Source: CAD feature listing. Evaluate the final solid. Frame: model axes, mm. A direction names the side the tool comes from. Give positions to 0.01 mm unless a question says otherwise; leave off trailing zeros. Loops run counter-clockwise (first coordinate to the right, second up) from the corner with the lowest first, then second, coordinate; pieces in that order, holes last. Notation, with made-up numbers: M -25,-9.5 L 3,-9.5 A21 ccw 3,14.5 Z; hole C -37.5,2 d4. An arc over 180 degrees is marked long. Write item = value, one per line.
Autodesk Inventor part; units mm, degrees
ref_plane "YZ Plane" through (0, 0, 0) normal (1, 0, 0) x (0, 1, 0)
ref_plane "XZ Plane" through (0, 0, 0) normal (0, 1, 0) x (-1, 0, 0)
ref_plane "XY Plane" through (0, 0, 0) normal (0, 0, 1) x (1, 0, 0)
sketch "Sketch1" plane through (0, 0, 0) normal (0, 1, 0) x (-1, 0, 0)
  circle A0 centre (0, 0) radius 6.125 construction
  circle A1 centre (0, 0) radius 6.825
  circle A2 centre (0, 0) radius 5.225
  circle A3 centre (0, 0) radius 5.425 construction
  line L0 (0, 0) -> (5.225, 0) construction
  line L1 (6.825, 0) -> (5.1994, 0) construction
  line L2 (6.125, 0) -> (6.825, 0) construction
  line L3 (5.425, 0) -> (6.125, 0) construction
  line L4 (5.225, 0) -> (5.425, 0) construction
  line L5 (5.361, -0.8306) -> (5.1634, -0.8)
  arc A4 (5.361, -0.8306) -> (6.8101, -0.45) centre (5.4797, 1.6666) ccw
  line L6 (5.361, 0.8306) -> (5.1634, 0.8)
  arc A5 (6.8101, 0.45) -> (5.361, 0.8306) centre (5.4797, -1.6666) ccw
  point P0 (5.1634, 0.8)
  point P1 (6.8101, 0.45)
  dimension "d0" = 12.25
  dimension "d1" = 0.7
  dimension "d2" = 0.7
  dimension "d3" = 0.2
  dimension "d4" = 0.8
  dimension "d5" = 2.5
  dimension "d6" = 0.45
extrude "Extrusion1" add sketch "Sketch1" along normal blind 10 contours A1 A4 L5 A2 L6 A5 | A2 picked at (5.9792, 0)
pattern_circular "Circular Pattern1" count 10 over 360 about axis through (0, 0, 0) along (0, 1, 0) of "Extrusion1"
sketch "Sketch3" plane through (0, 0, 0) normal (0, -1, 0) x (1, 0, 0)
  arc A0 (-4.6475, 2.3878) -> (-5.1634, 0.8) centre (0, 0) ccw construction
  circle A1 centre (0, 0) radius 2.5
  dimension "d13" = 5
extrude "Extrusion2" add sketch "Sketch3" along normal blind 3.75
properties part number "planeta_V2"
1. Cut plane C-C, the plane y = -1. Return the cut outline in (x, z).
Derived:
outline = C 0,0 d5
2. First-contact query: pin 1 Ø4 at (x, y) = (-1, 4.5) entering from -Z; pin 2 Ø3 at (y, z) = (0, 2) entering from -X; pin 3 Ø2 at (y, z) = (2, 1.5) entering from +X. Flat tips, straight axial feed; report the tip coordinate or a pass-through.
Derived:
pin_1 = -6.62
pin_2 = -6.73
pin_3 = 6.73
3. Reachability of faces 1 (the cylindrical face through (-2.115, 4.93, -6.489)), 2 (the cylindrical face through (5.4, 4.9, -3)), 3 (the cylindrical face through (-3.062, 4.93, 4.234)), 4 (the cylindrical face through (-4.5, 4.9, 4.2)), 5 (the cylindrical face through (-4.5, 4.9, -4.2)) from +Z, -Z, +X, -X, +Y, -Y: full face, straight path, thin tool, end or side. Return the list, or none.
Derived:
face_1 = -Z, -X, +Y, -Y
face_2 = +X, +Y, -Y
face_3 = +Y, -Y
face_4 = +Z, +Y, -Y
face_5 = -Z, +Y, -Y
4. Cut plane B-B, the plane z = 0. Return the cut outline in (x, y) (3 decimals).
Derived:
outline = M -6.825,0 L -2.5,0 L -2.5,-3.75 L 2.5,-3.75 L 2.5,0 L 6.825,0 L 6.825,10 L -6.825,10 Z
5. Cut plane A-A, the plane x = 0. Return the cut outline in (y, z) (3 decimals), then the cut area to 3 significant figures.
Derived:
outline = M -3.75,-2.5 L 0,-2.5 L 0,-5.225 L 10,-5.225 L 10,5.225 L 0,5.225 L 0,2.5 L -3.75,2.5 Z
area = 123 mm²
6. Pull-direction query (X, two-part tool) for faces 6 (the cylindrical face through (2.604, 4.93, 5.573)), 7 (the cylindrical face through (1.181, 4.93, 6.057)), 8 (the flat face through (0, 0, -3)); classes: +X half, -X half, draft (parallel to the pull), parting line (faces both ways), or undercut.
Derived:
face_6 = +X half
face_7 = undercut
face_8 = draft
7. Material intervals for probe 1 along Z at (x, y) = (-5.5, 9.75); probe 2 along X at (y, z) = (7.25, -4); probe 3 along Z at (x, y) = (-4.75, 6.5), sorted ascending. Write a range as from..to.
Derived:
probe_1 = -4.04..-3.13, -0.83..0.83, 3.13..4.04
probe_2 = -5.53..-4.1, -3.36..3.36, 4.1..5.53
probe_3 = -4.28..-2.44, -2.18..2.18, 2.44..4.28
